from build123d import *

# Parameters (mm, degrees)
SKETCH1_W               = 240
SKETCH1_H               = 20
BOSS_EXTRUDE1_DEPTH     = 30
SKETCH2_R               = 5.025
CUT_EXTRUDE1_DEPTH      = 20
SKETCH3_R               = 2.05
CUT_EXTRUDE2_DEPTH      = 30
CUT_EXTRUDE5_DEPTH      = 32.5
FILLET1_R               = 10
FILLET2_R               = 10
CHAMFER1_SIZE           = 1
CHAMFER2_SIZE           = 1
CUT_EXTRUDE9_DEPTH      = 3
CUT_EXTRUDE9_DEPTH_BACK = 3
SKETCH10_R              = 3.65
SKETCH11_R              = 1.5
CUT_EXTRUDE10_DEPTH     = 13
SKETCH12_R              = 2.75
SKETCH12_R_2            = 1.5
CUT_EXTRUDE11_DEPTH     = 3
SKETCH16_R              = 2.05
CUT_EXTRUDE12_DEPTH     = 40


with BuildPart() as part:
    # Sketch1 → Boss-Extrude1 (new body)
    with BuildSketch(Plane(origin=(0, 0, 0), x_dir=(0, 0, -1), z_dir=(1, 0, 0))):
        with Locations((47.599764496, 4.521643901)):
            Rectangle(SKETCH1_W, SKETCH1_H)
    extrude(amount=BOSS_EXTRUDE1_DEPTH)

    # Sketch2 → Cut-Extrude1 (cut)
    with BuildSketch(Plane(origin=(0, 14.521643901, 0), x_dir=(1, 0, 0), z_dir=(0, 1, 0))):
        with Locations(Location((15, 147.599764496, 0), (0, 0, 270))):
            Circle(SKETCH2_R)
        with Locations(Location((15, -52.400235504, 0), (0, 0, 270))):
            Circle(SKETCH2_R)
    extrude(amount=-CUT_EXTRUDE1_DEPTH, mode=Mode.SUBTRACT)

    # Sketch3 → Cut-Extrude2 (cut)
    with BuildSketch(Plane(origin=(30, 0, 0), x_dir=(0, 0, -1), z_dir=(1, 0, 0))):
        with Locations((117.599764496, 4.521643901)):
            Circle(SKETCH3_R)
        with Locations((-22.400235504, 4.521643901)):
            Circle(SKETCH3_R)
        with Locations((12.599764496, 4.521643901)):
            Circle(SKETCH3_R)
        with Locations((82.599764496, 4.521643901)):
            Circle(SKETCH3_R)
    extrude(amount=-CUT_EXTRUDE2_DEPTH, mode=Mode.SUBTRACT)

    # Sketch6 → Cut-Extrude5 (cut)
    with BuildSketch(Plane.XZ.offset(5.478356099)):
        Polygon((30, 37.400235504), (20, 25.482699578), (20, -14.517300422), (30, -26.434836348), align=None)
        Polygon((30, -68.764692644), (20, -80.68222857), (20, -120.68222857), (30, -132.599764496), align=None)
    extrude(amount=-CUT_EXTRUDE5_DEPTH, mode=Mode.SUBTRACT)

    # Fillet1
    fillet1_edges = [part.edges().sort_by_distance(p)[0] for p in [
        (30, 4.521643901, -26.434836348),
        (30, 4.521643901, -68.764692644),
    ]]
    fillet(fillet1_edges, radius=FILLET1_R)

    # Fillet2
    fillet2_edges = [part.edges().sort_by_distance(p)[0] for p in [
        (30, 4.521643901, 72.400235504),
        (30, 4.521643901, -167.599764496),
        (30, 4.521643901, 37.400235504),
        (30, 4.521643901, -132.599764496),
    ]]
    fillet(fillet2_edges, radius=FILLET2_R)

    # Chamfer1
    chamfer1_edges = [part.edges().sort_by_distance(p)[0] for p in [
        (30, -5.478356099, 51.720086675),
        (23.830222216, -5.478356099, 30.047380664),
        (10, -5.478356099, 72.400235504),
        (10, -5.478356099, -167.599764496),
        (30, -5.478356099, -146.919615667),
        (29.396926208, -5.478356099, 37.619736413),
        (29.396926208, -5.478356099, -132.819265405),
        (27.071067812, -5.478356099, -164.670832308),
        (27.071067812, -5.478356099, 69.471303316),
        (20, -5.478356099, 5.482699578),
        (23.830222216, -5.478356099, -19.081981508),
        (20, -5.478356099, -100.68222857),
        (23.830222216, -5.478356099, -125.246909656),
        (30, -5.478356099, -47.599764496),
        (23.830222216, -5.478356099, -76.117547484),
        (29.396926208, -5.478356099, -68.545191735),
        (29.396926208, -5.478356099, -26.654337257),
    ]]
    chamfer(chamfer1_edges, length=CHAMFER1_SIZE)

    # Chamfer2
    chamfer2_edges = [part.edges().sort_by_distance(p)[0] for p in [
        (29.396926208, 14.521643901, -26.654337257),
        (30, 14.521643901, 51.720086675),
        (10, 14.521643901, 72.400235504),
        (30, 14.521643901, -146.919615667),
        (10, 14.521643901, -167.599764496),
        (23.830222216, 14.521643901, 30.047380664),
        (29.396926208, 14.521643901, 37.619736413),
        (29.396926208, 14.521643901, -132.819265405),
        (27.071067812, 14.521643901, -164.670832308),
        (27.071067812, 14.521643901, 69.471303316),
        (23.830222216, 14.521643901, -19.081981508),
        (20, 14.521643901, 5.482699578),
        (23.830222216, 14.521643901, -125.246909656),
        (20, 14.521643901, -100.68222857),
        (30, 14.521643901, -47.599764496),
        (23.830222216, 14.521643901, -76.117547484),
        (29.396926208, 14.521643901, -68.545191735),
    ]]
    chamfer(chamfer2_edges, length=CHAMFER2_SIZE)

    # Sketch10 → Cut-Extrude9 (cut, two sides: drawn at the far end of the back side and taken through both)
    with BuildSketch(Plane(origin=(20, 0, 0), x_dir=(0, 0, -1), z_dir=(1, 0, 0)).offset(-CUT_EXTRUDE9_DEPTH_BACK)):
        with Locations(Location((12.599764496, 4.521643901, 0), (0, 0, 301.691963515))):
            Circle(SKETCH10_R)
        with Locations(Location((-22.400235504, 4.521643901, 0), (0, 0, 147.61954983))):
            Circle(SKETCH10_R)
        with Locations(Location((82.599764496, 4.521643901, 0), (0, 0, 238.308036485))):
            Circle(SKETCH10_R)
        with Locations(Location((117.599764496, 4.521643901, 0), (0, 0, 327.61954983))):
            Circle(SKETCH10_R)
    extrude(amount=CUT_EXTRUDE9_DEPTH + CUT_EXTRUDE9_DEPTH_BACK, mode=Mode.SUBTRACT)

    # Sketch11 → Cut-Extrude10 (cut)
    with BuildSketch(Plane(origin=(30, 0, 0), x_dir=(0, 0, -1), z_dir=(1, 0, 0))):
        with Locations((147.599764496, 4.521643901)):
            Circle(SKETCH11_R)
        with Locations((-52.400235504, 4.521643901)):
            Circle(SKETCH11_R)
    extrude(amount=-CUT_EXTRUDE10_DEPTH, mode=Mode.SUBTRACT)

    # Sketch12 → Cut-Extrude11 (cut)
    # profile 1 of 2: a face of its own
    with BuildSketch(Plane(origin=(30, 0, 0), x_dir=(0, 0, -1), z_dir=(1, 0, 0))):
        with Locations((-52.400235504, 4.521643901)):
            Circle(SKETCH12_R)
        with Locations((-52.400235504, 4.521643901)):
            Circle(SKETCH12_R_2, mode=Mode.SUBTRACT)
    # profile 2 of 2: a face of its own
    with BuildSketch(Plane(origin=(30, 0, 0), x_dir=(0, 0, -1), z_dir=(1, 0, 0))):
        with Locations((147.599764496, 4.521643901)):
            Circle(SKETCH12_R)
        with Locations((147.599764496, 4.521643901)):
            Circle(SKETCH12_R_2, mode=Mode.SUBTRACT)
    extrude(amount=-CUT_EXTRUDE11_DEPTH, mode=Mode.SUBTRACT)

    # Sketch16 → Cut-Extrude12 (cut)
    with BuildSketch(Plane(origin=(0, 14.521643901, 0), x_dir=(1, 0, 0), z_dir=(0, 1, 0))):
        with Locations(Location((10, 77.599764496, 0), (0, 0, 270))):
            Circle(SKETCH16_R)
        with Locations(Location((10, 17.599764496, 0), (0, 0, 270))):
            Circle(SKETCH16_R)
    extrude(amount=-CUT_EXTRUDE12_DEPTH, mode=Mode.SUBTRACT)


solid = part.part
Design review of the part built by this model. Coordinates are the model's own, in mm. A direction names the side the tool comes from. Coordinates: 2 decimals unless noted, no trailing zeros. Loops run counter-clockwise (first coordinate to the right, second up) from the corner with the lowest first, then second, coordinate; pieces in that order, holes last. Notation, with made-up numbers: M -37.5,30 L 2.5,30 A18 ccw 2.5,45 Z; hole C 24.5,-6 d9. An arc over 180 degrees is marked long. Answer as CSV lines item,"result".
Item 1: The part is to be moulded in two halves that separate along Y. For faces 6 (the face through (23.391, -4.971, -75.874)), 7 (the face through (20, 4, 6)), 8 (the face through (26.56, 14.35, -164.01)), 9 (the face through (17, 2, -12)), say which applies: pulls with the +Y half, pulls with the -Y half, needs draft (parallel to the pull), parting line crosses it, or undercut.
Answer list:
face 6,"pulls with the -Y half"
face 7,"needs draft"
face 8,"pulls with the +Y half"
face 9,"undercut"
Item 2: For probe 1 along Z at (x, y) = (5.5, 4.5); probe 2 along Z at (x, y) = (11.5, -0.75); probe 3 along Z at (x, y) = (24, 9), list the stretches that pass through material, from the lowest coordinate up.
Answer list:
probe 1,"-167.6 to -119.65, -115.55 to -84.65, -80.55 to -14.65, -10.55 to 20.35, 24.45 to 72.4"
probe 2,"-167.6 to -151.21, -143.99 to -79, -76.2 to -19, -16.2 to 48.79, 56.01 to 72.4"
probe 3,"-166.76 to -125.45, -75.92 to -19.28, 30.25 to 71.57"
Item 3: Add section B-B on z = -89. State the section outline as (x, y) points.
Answer list:
outline,"M 0,-5.48 L 19,-5.48 L 20,-4.48 L 20,13.52 L 19,14.52 L 0,14.52 Z"
Item 4: Machinability: for faces 1 (the face through (23.39, -4.97, 30.29)), 2 (the face through (20, 4, -100)), 3 (the face through (18.749, 3.583, -121.127)), 4 (the face through (0, 5, -46)), 5 (the face through (10, 4, 72.4)), which of the approach directions +Z, -Z, +X, -X, +Y, -Y give a long, thin tool a straight path to every point of the face, cutting with its end or side? Answer none if there is none.
Answer list:
face 1,"+X, -Y"
face 2,"+X, +Y, -Y"
face 3,"+X"
face 4,"+Z, -Z, -X, +Y, -Y"
face 5,"+Z, +X, -X, +Y, -Y"
Item 5: For P1, Ø9, axis at y = 3, z = 9.5, coming from the +X side; P2, Ø6.5, axis at y = 4.52, z = 22.4, coming from the +X side; P3, Ø1.5, axis at x = 23, y = 1, coming from the +Z side, all flat-tipped, find the tip position at first contact; note any pin that passes through.
Answer list:
P1,"x = 20"
P2,"x = 17"
P3,"z = 72.14"
Item 6: Add section A-A on x = 15. State the section outline as (y, z) points, plus the area to 3 significant figures.
Answer list:
outline,"M -5.48,-166.6 L -4.48,-167.6 L 13.52,-167.6 L 14.52,-166.6 L 14.52,-152.62 L -5.48,-152.62 Z; M -5.48,-142.57 L 14.52,-142.57 L 14.52,47.38 L -5.48,47.38 Z; M -5.48,57.43 L 14.52,57.43 L 14.52,71.4 L 13.52,72.4 L -4.48,72.4 L -5.48,71.4 Z; hole C 4.52,-117.6 d4.1; hole C 4.52,-82.6 d4.1; hole C 4.52,-12.6 d4.1; hole C 4.52,22.4 d4.1"
area,"4,340 mm²"
